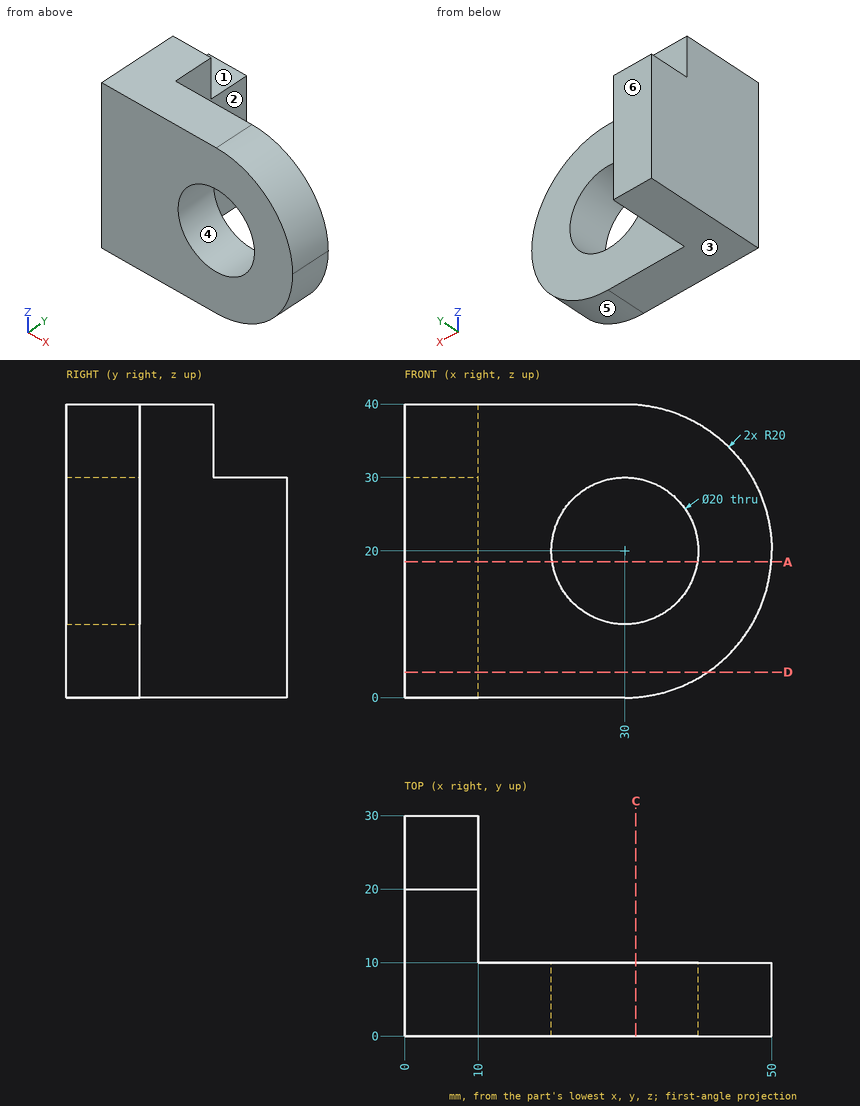
Part print with two shaded views. Sizes in mm from the minimum x, y, z corner. A direction names the side the tool comes from. Round coordinates to 2 decimals unless told otherwise and drop trailing zeros. Order: outer loops, then holes, each group sorted by start corner. A loop starts at its lowest first (then second) coordinate and runs counter-clockwise, first axis right, second up.
(1) Drill centre lines: line 1 (X direction, y = 5, z = 20); line 2 (Z direction, x = 30, y = 7.75); line 3 (Y direction, x = 39, z = 9). Where is each one in solid material? Low to high.
(2) 3-axis set-ups, long thin cutter, end or side, ignore diameter. For the marked faces 1, 2 and 3: which of +Z, -Z, +X, -X, +Y, -Y reach the whole face in a straight line?
(3) Band-saw the part on A-A (z = 18.5). List the corners of the cut face in (x, y).
(4) Band-saw the part on D-D (z = 3.5). List the corners of the cut face in (x, y), then the cut area to 3 significant figures.
(5) Pin check, flat tips, straight feed: pin 1 (3 mm diameter, centred on y = 22.5, z = 26.5, fed in from -X); pin 2 (23 mm diameter, centred on x = 30, z = 20, fed in from +Y); pin 3 (5 mm diameter, centred on x = 6.5, y = 23.5, fed in from +Z); pin 4 (10 mm diameter, centred on y = 21.5, z = 23, fed in from +X). Stop position of each tip, or through.
(6) Band-saw the part on C-C (x = 31.5). List the corners of the cut face in (y, z), then the cut area to 3 significant figures.
(7) Pull direction Z, two halves, no side cores. Call the marked faces 4, 5 and 6: released by +Z, released by -Z, zero draft, split by the parting line, or undercut.
Verdict:
1. line 1: x = 0 to 20, 40 to 50
1. line 2: z = 0 to 10, 30 to 40
1. line 3: y = 0 to 10
2. face 1: +Z, +X, -X, +Y
2. face 2: +Z, -Z, +X, +Y
2. face 3: -Z, +X, -X, +Y, -Y
3. outline: (0, 0) - (20.11, 0) - (20.11, 10) - (10, 10) - (10, 30) - (0, 30) - close; (39.89, 0) - (49.94, 0) - (49.94, 10) - (39.89, 10) - close
4. outline: (0, 0) - (41.3, 0) - (41.3, 10) - (10, 10) - (10, 30) - (0, 30) - close
4. area: 613 mm2
5. pin 1: stops at x = 0
5. pin 2: stops at y = 10
5. pin 3: stops at z = 30
5. pin 4: stops at x = 10
6. outline: (0, 0.06) - (10, 0.06) - (10, 10.11) - (0, 10.11) - close; (0, 29.89) - (10, 29.89) - (10, 39.94) - (0, 39.94) - close
6. area: 201 mm2
7. face 4: undercut
7. face 5: released by -Z
7. face 6: zero draft
